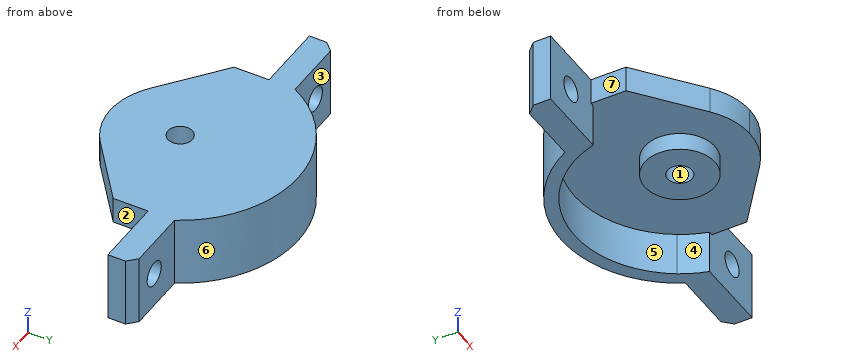
Autodesk Inventor part; units mm, degrees
ref_plane "YZ Plane" through (0, 0, 0) normal (1, 0, 0) x (0, 1, 0)
ref_plane "XZ Plane" through (0, 0, 0) normal (0, 1, 0) x (-1, 0, 0)
ref_plane "XY Plane" through (0, 0, 0) normal (0, 0, 1) x (1, 0, 0)
sketch "Эскиз1" plane through (0, 0, 0) normal (0, 0, 1) x (1, 0, 0)
  circle A0 centre (0, 0) radius 10.75 construction
  line L0 (-40.1576, -0.75) -> (35.328, -0.75) construction
  line L1 (-40.1576, 3.25) -> (35.328, 3.25) construction
  line L2 (-12, 3.25) -> (-20, 3.25)
  line L3 (-20, 3.25) -> (-20, 6.25)
  line L4 (-20, 6.25) -> (0, 6.25)
  line L5 (0, 6.25) -> (0, -8)
  arc A1 (-4.9401, -6.2925) -> (0, -8) centre (0, 0) ccw
  line L6 (12, 3.25) -> (20, 3.25)
  line L7 (20, 3.25) -> (20, 6.25)
  line L8 (20, 6.25) -> (0, 6.25)
  arc A2 (0, -8) -> (4.9401, -6.2925) centre (0, 0) ccw
  line L9 (12, 3.25) -> (12, -0.75)
  line L10 (-12, 3.25) -> (-12, -0.75)
  line L11 (-4.9401, -6.2925) -> (-12, -0.75)
  line L12 (4.9401, -6.2925) -> (12, -0.75)
  dimension "d1" = 21.5
  dimension "d2" = 0.75
  dimension "d3" = 4
  dimension "d4" = 8
  dimension "d5" = 3
  dimension "d6" = 24
  dimension "d7" = 40
extrude "Выдавливание1" add sketch "Эскиз1" along normal blind 3
sketch "Эскиз2" plane through (0, 0, 0) normal (0, 0, -1) x (-1, 0, 0)
  arc A0 (-4.9401, -6.2925) -> (4.9401, -6.2925) centre (0, 0) ccw
  circle A1 centre (0, 0) radius 4
  line L0 (-20, 6.25) -> (20, 6.25)
  line L1 (-12, 3.25) -> (-20, 3.25)
  line L2 (-20, 3.25) -> (-20, 6.25)
  line L3 (-11.5515, 3.25) -> (-20, 3.25)
  line L4 (-20, 3.25) -> (-20, 6.25)
  line L5 (-20, 6.25) -> (-10.2439, 6.25)
  line L6 (10.2439, 6.25) -> (20, 6.25)
  line L7 (20, 6.25) -> (20, 3.25)
  line L8 (20, 6.25) -> (20, 3.25)
  line L9 (20, 3.25) -> (11.5515, 3.25)
  arc A2 (-10.2439, 6.25) -> (-11.5515, 3.25) centre (0, 0) ccw
  arc A3 (11.5515, 3.25) -> (10.2439, 6.25) centre (0, 0) ccw
  line L10 (-20, 6.25) -> (20, 6.25)
  dimension "d10" = 8
  dimension "d26" = 12
extrude "Выдавливание2" add sketch "Эскиз2" along normal blind 2
sketch "Эскиз3" plane through (0, 0, -2) normal (0, 0, -1) x (-1, 0, 0)
  line L0 (-10.2439, 6.25) -> (-20, 6.25)
  line L1 (-20, 6.25) -> (-20, 3.25)
  line L2 (-20, 3.25) -> (-11.5515, 3.25)
  line L3 (11.5515, 3.25) -> (20, 3.25)
  line L4 (20, 3.25) -> (20, 6.25)
  arc A0 (11.5515, 3.25) -> (10.2439, 6.25) centre (0, 0) ccw
  line L5 (20, 6.25) -> (10.2439, 6.25)
  arc A1 (-10.2439, 6.25) -> (-11.5515, 3.25) centre (0, 0) ccw
extrude "Выдавливание3" add sketch "Эскиз3" along normal blind 3
sketch "Эскиз4" plane through (0, 0, -2) normal (0, 0, -1) x (-1, 0, 0)
  circle A0 centre (0, 0) radius 4
hole "Отверстие1" at (0, 0, -2) direction (0, 0, 1) diameter 2.8 end through all
sketch "Эскиз5" plane through (0, 0, 3) normal (0, 0, 1) x (1, 0, 0)
  arc A0 (10.2439, 6.25) -> (-10.2439, 6.25) centre (0, 0) ccw
  line L0 (20, 6.25) -> (-20, 6.25)
  arc A1 (11.9661, 6.25) -> (-11.9661, 6.25) centre (0, 0) ccw
  line L1 (11.9661, 6.25) -> (10.2439, 6.25)
  line L2 (-10.2439, 6.25) -> (-11.9661, 6.25)
  dimension "d22" = 12
  dimension "d23" = 1.5
extrude "Выдавливание4" add sketch "Эскиз5" against normal up to surface (8 mm away) contours A0 L0 A1
sketch "Эскиз6" plane through (0, 0, 3) normal (0, 0, 1) x (1, 0, 0)
  arc A0 (10.2439, 6.25) -> (-10.2439, 6.25) centre (0, 0) ccw
  line L0 (10.2439, 6.25) -> (-10.2439, 6.25)
extrude "Выдавливание5" add sketch "Эскиз6" against normal up to surface (3 mm away)
sketch "Эскиз7" plane through (20, 6.25, 3) normal (0, 1, 0) x (1, 0, 0)
  line L0 (-40, 8) -> (-40, 0)
  line L1 (-31.5515, 8) -> (-8.4485, 8)
  line L2 (-20, 8) -> (-20, 0)
  line L3 (-24.9401, 0) -> (-15.0599, 0)
  point P0 (-20, 3)
  point P1 (-4, 4)
  point P2 (-36, 4)
  point P3 (-40, 4)
  dimension "d36" = 32
hole "Отверстие2" at (16, 6.25, -1) at (-16, 6.25, -1) direction (0, -1, 0) diameter 2.8 end through all
chamfer "Фаска1" distance 1 angle 45 2 edges at (20, 6.25, -1) (-20, 6.25, -1)
properties part number "smallWheelStator" material "Пластик АБС"
Here's how the part is built. I have some questions about the finished solid (model axes, mm). Face numbers are marked on the shaded views. A direction names the side the tool comes from. Round coordinates to 2 decimals unless told otherwise and drop trailing zeros. Write each loop counter-clockwise with the first axis right and the second up, starting at its lowest first coordinate (ties: lowest second). Pieces come first, ordered by that corner, then holes.
1. Suppose I cut it at C-C (x = -11). List the corners of the cut face in (y, z) for me, and give its area (3 significant figures).
2. I need wall thicknesses on L1, parallel to Y at x = 0, z = -0.85; L2, parallel to X at y = 0, z = 1.5; L3, parallel to X at y = 4.5, z = -1. Which ranges of each line are inside material? Lowest first, please.
3. Suppose I cut it at D-D (y = 10.5). List the corners of the cut face in (x, z) for me, and give its area (3 significant figures).
4. Suppose I cut it at B-B (y = -3.5). List the corners of the cut face in (x, z) for me.
5. If we mould it in two halves opening along X, with no side actions, what happens to the marked faces 1, 2 and 3? For each: released by +X, released by -X, zero draft, split by the parting line, or undercut.
6. Suppose I cut it at A-A (x = 16). List the corners of the cut face in (y, z) for me, and give its area (3 significant figures).
7. Will these pins go through, and if not, where does the flat tip stop? pin 1 Ø4 at (x, z) = (-16.5, -1.5) entering from -Y; pin 2 Ø2.5 at (y, z) = (0.5, 1.5) entering from -X; pin 3 Ø1.7 at (x, z) = (16, -1) entering from -Y; pin 4 Ø6.5 at (x, y) = (-0.5, 0.5) entering from -Z.
8. For the marked faces 4, 5, 6 and 7, which set-ups out of +Z, -Z, +X, -X, +Y, -Y let a thin tool reach every point of the face, with its end or its side?
Answer sheet:
1. outline: (-1.54, 0) - (4.8, 0) - (4.8, -5) - (7.83, -5) - (7.83, 3) - (-1.54, 3) - close
1. area: 43.2 mm2
2. L1: y = -4 to -1.4, 1.4 to 4, 12 to 13.5
2. L2: x = -12 to -1.4, 1.4 to 12
2. L3: x = -20 to -17.4, -14.6 to -11.12, 11.12 to 14.6, 17.4 to 20
3. outline: (-8.49, -5) - (-5.81, -5) - (-5.81, 0) - (5.81, 0) - (5.81, -5) - (8.49, -5) - (8.49, 3) - (-8.49, 3) - close
3. area: 77.7 mm2
4. outline: (-8.5, 0) - (-1.94, 0) - (-1.94, -2) - (1.94, -2) - (1.94, 0) - (8.5, 0) - (8.5, 3) - (-8.5, 3) - close
5. face 1: undercut
5. face 2: released by +X
5. face 3: zero draft
6. outline: (3.25, -5) - (6.25, -5) - (6.25, -2.4) - (3.25, -2.4) - close; (3.25, 0.4) - (6.25, 0.4) - (6.25, 3) - (3.25, 3) - close
6. area: 15.6 mm2
7. pin 1: stops at y = 3.25
7. pin 2: stops at x = -12
7. pin 3: passes through
7. pin 4: stops at z = -2
8. face 4: -Z, -Y
8. face 5: -Z
8. face 6: +Z, -Z, +Y
8. face 7: +Z, -Z, -X, -Y
